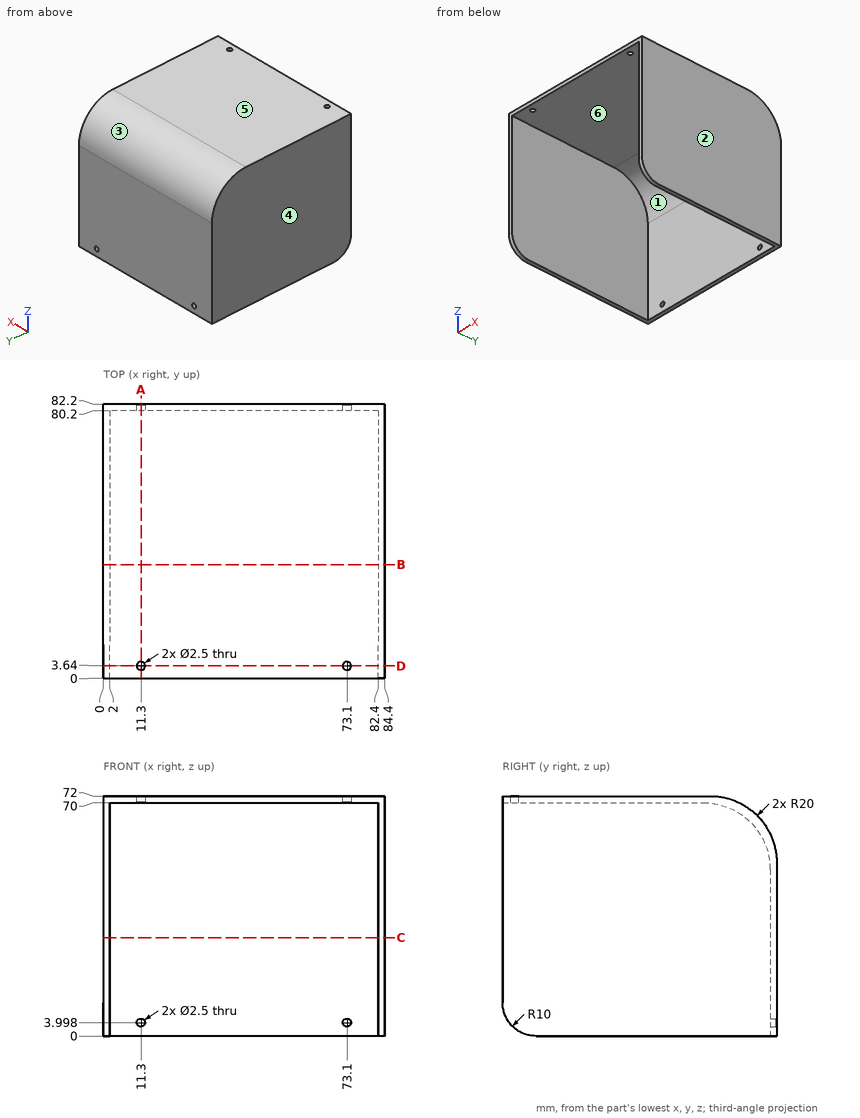
The figure shows three views and two pictorial views of one solid part (mm, origin at its lowest corner). Answer the questions. A direction names the side the tool comes from. Coordinates: 2 decimals unless noted, no trailing zeros. Loops run counter-clockwise (first coordinate to the right, second up) from the corner with the lowest first, then second, coordinate; pieces in that order, holes last. Notation, with made-up numbers: (53.25, -6) - (95.25, -6) arc R18 ccw to (95.25, -1) - close; hole circle Ø6 at (14.5, 68). An arc over 180 degrees is marked (long way). Answer in a Markdown table with one row per item.
Q1. The mould has two halves that part along X. Classify the marked faces 1, 2, 3 and 4: pulls with the +X half, pulls with the -X half, needs draft (parallel to the pull), parting line crosses it, or undercut.
Here are the results:
| item | result |
|---|---|
| face 1 | undercut |
| face 2 | pulls with the +X half |
| face 3 | needs draft |
| face 4 | pulls with the -X half |
Q2. Find section A-A on x = 11.3. Write down the section's boundary in (y, z), plus the area to 3 significant figures.
Here are the results:
| item | result |
|---|---|
| outline | (0, 70) - (2.39, 70) - (2.39, 72) - (0, 72) - close; (4.89, 70) - (60.2, 70) arc R20 cw to (80.2, 50) - (80.2, 5.25) - (82.2, 5.25) - (82.2, 52) arc R20 ccw to (62.2, 72) - (4.89, 72) - close; (80.2, 0) - (82.2, 0) - (82.2, 2.75) - (80.2, 2.75) - close |
| area | 294 mm^2 |
Q3. Find section C-C on z = 29.5. Write down the section's boundary in (x, y).
Here are the results:
| item | result |
|---|---|
| outline | (0, 0) - (2, 0) - (2, 80.2) - (82.4, 80.2) - (82.4, 0) - (84.4, 0) - (84.4, 82.2) - (0, 82.2) - close |
Q4. Given P1, Ø1.5, axis at x = 73.1, z = 4, coming from the -Y side; P2, Ø3, axis at x = 59, z = 13.5, coming from the -Y side; P3, Ø6, axis at x = 55, z = 55.5, coming from the -Y side, each flat-ended and moving along its own axis, determine where each tip first touches the part or whether it passes through.
Here are the results:
| item | result |
|---|---|
| P1 | passes through |
| P2 | stops at y = 80.2 |
| P3 | stops at y = 78.3 |
Q5. Find section D-D on y = 3.64. Write down the section's boundary in (x, z), plus the area to 3 significant figures.
Here are the results:
| item | result |
|---|---|
| outline | (0, 2.28) - (2, 2.28) - (2, 70) - (10.05, 70) - (10.05, 72) - (0, 72) - close; (12.55, 70) - (71.85, 70) - (71.85, 72) - (12.55, 72) - close; (74.35, 70) - (82.4, 70) - (82.4, 2.28) - (84.4, 2.28) - (84.4, 72) - (74.35, 72) - close |
| area | 430 mm^2 |
Q6. Find section B-B on y = 34. Write down the section's boundary in (x, z).
Here are the results:
| item | result |
|---|---|
| outline | (0, 0) - (2, 0) - (2, 70) - (82.4, 70) - (82.4, 0) - (84.4, 0) - (84.4, 72) - (0, 72) - close |
Q7. Straight lines are drawn through the part: line 1 along X through (y, z) = (75, 27); line 2 along X through (y, z) = (3, 71); line 3 along Z through (x, y) = (34, 54). For each, find the intervals that lie inside material, in ascending order. Write a range as [from, to].
Here are the results:
| item | result |
|---|---|
| line 1 | x = [0, 2], [82.4, 84.4] |
| line 2 | x = [0, 10.23], [12.37, 72.03], [74.17, 84.4] |
| line 3 | z = [70, 72] |
Q8. For the marked faces 5 and 6, determine the directions among +Z, -Z, +X, -X, +Y, -Y from which every point of the face is accessible in a straight line to the end or side of a thin tool.
Here are the results:
| item | result |
|---|---|
| face 5 | +Z, +X, -X, +Y, -Y |
| face 6 | -Z, -Y |
